Read the model definition and answer for the solid it produces. Units are mm, in the model's axes. A direction names the side the tool comes from. Round coordinates to 2 decimals unless told otherwise and drop trailing zeros. Write each loop counter-clockwise with the first axis right and the second up, starting at its lowest first coordinate (ties: lowest second). Pieces come first, ordered by that corner, then holes.
from build123d import *

# Parameters (mm, degrees)
SKETCH1_W               = 50
SKETCH1_H               = 35
BOSS_EXTRUDE1_DEPTH     = 8
CUT_EXTRUDE1_DEPTH      = 1
CUT_EXTRUDE1_DEPTH_BACK = 51
FILLET1_R               = 2
SKETCH5_W               = 35
SKETCH5_H               = 2
BOSS_EXTRUDE2_DEPTH     = 10
SKETCH6_R               = 1.5
CUT_EXTRUDE2_DEPTH      = 10
SKETCH3_W               = 10
SKETCH3_H               = 2
CUT_EXTRUDE3_DEPTH      = 36
FILLET3_R               = 5


with BuildPart() as part:
    # Sketch1 → Boss-Extrude1 (new body)
    with BuildSketch(Plane(origin=(0, 0, 0), x_dir=(1, 0, 0), z_dir=(0, 1, 0))):
        Rectangle(SKETCH1_W, SKETCH1_H)
    extrude(amount=-BOSS_EXTRUDE1_DEPTH)

    # Sketch2 → Cut-Extrude1 (cut, two sides)
    with BuildSketch(Plane(origin=(25, 0, 0), x_dir=(0, 0, -1), z_dir=(1, 0, 0))) as cut_extrude1_sk:
        Polygon((-12.5, -5), (-17.5, -8), (0, -8), (0, -5), align=None)
        Polygon((0, -5), (0, -8), (17.5, -8), (12.5, -5), align=None)
    extrude(amount=CUT_EXTRUDE1_DEPTH, mode=Mode.SUBTRACT)
    extrude(cut_extrude1_sk.sketch, amount=-CUT_EXTRUDE1_DEPTH_BACK, mode=Mode.SUBTRACT)

    # Fillet1
    fillet1_edges = [part.edges().sort_by_distance(p)[0] for p in [
        (0, -8, -17.5),
        (0, -5, 12.5),
        (0, -5, -12.5),
        (0, -8, 17.5),
    ]]
    fillet(fillet1_edges, radius=FILLET1_R)

    # Sketch5 → Boss-Extrude2 (add)
    with BuildSketch(Plane.ZY.offset(25)):
        with Locations((0, -1)):
            Rectangle(SKETCH5_W, SKETCH5_H)
    boss_extrude2 = extrude(amount=BOSS_EXTRUDE2_DEPTH)

    # Mirror1: Boss-Extrude2 across plane
    add(boss_extrude2.mirror(Plane(origin=(0, 0, 0), x_dir=(0, 0, 1), z_dir=(1, 0, 0))))

    # Sketch6 → Cut-Extrude2 (cut)
    with BuildSketch(Plane(origin=(0, 0, 0), x_dir=(1, 0, 0), z_dir=(0, 1, 0))):
        with Locations((-30, 14)):
            Circle(SKETCH6_R)
        with Locations((-30, -14)):
            Circle(SKETCH6_R)
        with Locations((30, -14)):
            Circle(SKETCH6_R)
        with Locations((30, 14)):
            Circle(SKETCH6_R)
    extrude(amount=-CUT_EXTRUDE2_DEPTH, mode=Mode.SUBTRACT)

    # Sketch3 → Cut-Extrude3 (cut, through all)
    with BuildSketch(Plane.XY.offset(17.5)):
        with Locations((5, -1)):
            Rectangle(SKETCH3_W, SKETCH3_H)
        with Locations((-5, -1)):
            Rectangle(SKETCH3_W, SKETCH3_H)
    extrude(amount=-CUT_EXTRUDE3_DEPTH, mode=Mode.SUBTRACT)

    # Fillet3
    fillet3_edges = [part.edges().sort_by_distance(p)[0] for p in [
        (-35, -1, -17.5),
        (-35, -1, 17.5),
        (35, -1, -17.5),
        (35, -1, 17.5),
    ]]
    fillet(fillet3_edges, radius=FILLET3_R)


solid = part.part
Q1. Section B-B (x = 0) is taken. Determine the outline of the cut face in (y, z), then the cut area to 3 significant figures.
Verdict:
outline: (-6.18, -14.47) arc R2 ccw to (-4.47, -17.5) - (-2, -17.5) - (-2, 17.5) - (-4.47, 17.5) arc R2 ccw to (-6.18, 14.47) - (-5.29, 12.98) arc R2 cw to (-5, 11.95) - (-5, -11.95) arc R2 cw to (-5.29, -12.98) - close
area: 114 mm2
Q2. Section D-D (x = 23.5) is taken. Determine the outline of the cut face in (y, z).
Verdict:
outline: (-6.18, -14.47) arc R2 ccw to (-4.47, -17.5) - (0, -17.5) - (0, 17.5) - (-4.47, 17.5) arc R2 ccw to (-6.18, 14.47) - (-5.29, 12.98) arc R2 cw to (-5, 11.95) - (-5, -11.95) arc R2 cw to (-5.29, -12.98) - close
Q3. Which of the six approach directions +Z, -Z, +X, -X, +Y, -Y give full straight-line access (tool end or side, diameter ignored) to faces 4 (the flat face through (-25, -4, 0)), 5 (the flat face through (-10, -1, 0)), 6 (the cylindrical face through (-31.5, -0.99, 13.93)), 7 (the flat face through (25, -4, 0)), 8 (the flat face through (0, -5, 0))?
Verdict:
face 4: +Z, -Z, -X, -Y
face 5: +Z, -Z, +Y
face 6: +Y, -Y
face 7: +Z, -Z, +X, -Y
face 8: +X, -X, -Y
Q4. Straight lines are drawn through the part: probe 1 along Z at (x, y) = (-30, -1); probe 2 along X at (y, z) = (-0.7, 14); probe 3 along Y at (x, z) = (32, -6). For each, find the intervals that lie inside material, in ascending order.
Verdict:
probe 1: z = -17.5 to -15.5, -12.5 to 12.5, 15.5 to 17.5
probe 2: x = -34.77 to -31.5, -28.5 to -10, 10 to 28.5, 31.5 to 34.77
probe 3: y = -2 to 0
Q5. Flat-ended cylindrical pins translate along their axes: pin 1 Ø6 at (x, z) = (-2.5, -2) entering from +Y; pin 2 Ø8 at (x, z) = (30.5, -3) entering from -Y; pin 3 Ø1.8 at (x, z) = (-30, 14) entering from +Y; pin 4 Ø3.5 at (y, z) = (-5, -1.5) entering from -X. Find the tip coordinate at first contact, or state that the pin passes through.
Verdict:
pin 1: stops at y = -2
pin 2: stops at y = -2
pin 3: passes through
pin 4: stops at x = -25
Q6. Section A-A (y = -1) is taken. Determine the outline of the cut face in (x, z).
Verdict:
outline: (-35, -12.5) arc R5 ccw to (-30, -17.5) - (-10, -17.5) - (-10, 17.5) - (-30, 17.5) arc R5 ccw to (-35, 12.5) - close; (10, -17.5) - (30, -17.5) arc R5 ccw to (35, -12.5) - (35, 12.5) arc R5 ccw to (30, 17.5) - (10, 17.5) - close; hole circle Ø3 at (-30, -14); hole circle Ø3 at (-30, 14); hole circle Ø3 at (30, -14); hole circle Ø3 at (30, 14)
Q7. Section C-C (z = 5) is taken. Determine the outline of the cut face in (x, y).
Verdict:
outline: (-35, -2) - (-25, -2) - (-25, -5) - (25, -5) - (25, -2) - (35, -2) - (35, 0) - (10, 0) - (10, -2) - (-10, -2) - (-10, 0) - (-35, 0) - close
Q8. Determine the mould class of faces 1 (the cylindrical face through (0.4, -6.2, -16.5)), 2 (the cylindrical face through (-33.57, -0.99, 16)), 3 (the flat face through (-35, -1, 0)) for opening direction Z: pulls with the +Z half, pulls with the -Z half, needs draft (parallel to the pull), parting line crosses it, or undercut.
Verdict:
face 1: undercut
face 2: pulls with the +Z half
face 3: needs draft
